```python
from build123d import *

# Parameters (mm, degrees)
F0_R      = 45.251608
F1_DEPTH  = 25.4
F1_FACE_R = 45.251608
F2_DEPTH  = 25.4
F4_D      = 50.8


with BuildPart() as f1:
    # F0 (on Top) → F1 (new body)
    with BuildSketch(Plane.XY):
        Circle(F0_R)
    extrude(amount=F1_DEPTH)

    # F1_face (on face) → F2 (join)
    with BuildSketch(Plane.XY.offset(25.4)):
        Circle(F1_FACE_R)
    extrude(amount=F2_DEPTH)

    # F4 (through all)
    with Locations(Plane.XY.offset(50.8)):
        with Locations((-29.471625, 2.728854), (28.161775, 0)):
            Hole(F4_D / 2)


solid = f1.part
```
Could you check a few things on this model? Use its own coordinates, in mm. Coordinates: 2 decimals unless noted, no trailing zeros. Write each loop counter-clockwise with the first axis right and the second up, starting at its lowest first coordinate (ties: lowest second). Pieces come first, ordered by that corner, then holes. Notation, with made-up numbers: (9, 25) -> (51, 25) arc R26 ccw to (51, 47) -> close; hole circle Ø6 at (78, -17). An arc over 180 degrees is marked (long way). Return JSON: item names as keys, results as strings.
(1) I need wall thicknesses on L1, parallel to Y at x = 14.5, z = 12.5; L2, parallel to Y at x = -26, z = 25; L3, parallel to X at y = -38, z = 44.5. Which ranges of each line are inside material? Lowest first, please.
Numbers:
{"L1": "y = -42.87 to -21.41, 21.41 to 42.87", "L2": "y = -37.04 to -22.43, 27.89 to 37.04", "L3": "x = -24.57 to 24.57"}
(2) Imagine slicing it at B-B, the plane x = -21. Please give me the cut outline in (y, z).
Numbers:
{"outline": "(-40.08, 0) -> (-21.22, 0) -> (-21.22, 50.8) -> (-40.08, 50.8) -> close; (26.67, 0) -> (40.08, 0) -> (40.08, 50.8) -> (26.67, 50.8) -> close"}
(3) Imagine slicing it at D-D, the plane z = 9.5. Please give me the cut outline in (x, y).
Numbers:
{"outline": "(-40.52, -20.14) arc R45.25 ccw to (38.98, -22.98) arc R25.4 cw (long way) to (38.98, 22.98) arc R45.25 ccw to (-36.13, 27.24) arc R25.4 cw (long way) to start"}
(4) Imagine slicing it at C-C, the plane y = 30.5. Please give me the cut outline in (x, z), then the cut area to 3 significant figures.
Numbers:
{"outline": "(-33.43, 0) -> (33.43, 0) -> (33.43, 50.8) -> (-33.43, 50.8) -> close", "area": "3,400 mm2"}
(5) I'm going to push flat-ended pins straight in: pin 1 (1 mm diameter, centred on x = 25.5, z = 10, fed in from -Y); pin 2 (1.5 mm diameter, centred on y = 13.5, z = 14, fed in from -X); pin 3 (10 mm diameter, centred on x = -26.5, z = 37, fed in from +Y). Where does each tip first touch, or does it pass through?
Numbers:
{"pin 1": "stops at y = -37.72", "pin 2": "stops at x = -6.83", "pin 3": "stops at y = 39.82"}
(6) Imagine slicing it at A-A, the plane x = 32.5. Please give me the cut outline in (y, z), then the cut area to 3 significant figures.
Numbers:
{"outline": "(-31.49, 0) -> (-25.03, 0) -> (-25.03, 50.8) -> (-31.49, 50.8) -> close; (25.03, 0) -> (31.49, 0) -> (31.49, 50.8) -> (25.03, 50.8) -> close", "area": "656 mm2"}
